```python
from build123d import *

# Parameters (mm, degrees)
FILLET1_R = 1


# Read off the part's stored shape, not the designer's step: Dog Bowl Washer
with BuildPart() as part:
    # Dog Bowl Washer outline → Dog Bowl Washer (revolve)
    with BuildSketch(Plane.XY):
        with BuildLine():
            Line((5.2705, 1.27), (6.392427617, 0))
            Line((6.392427617, 0), (12.7, 0))
            Line((12.7, 0), (12.646813167, 1.52307162))
            ThreePointArc((12.646813167, 1.52307162), (11.484828724, 4.047470654), (8.87095, 4.9911))
            Line((8.87095, 4.9911), (5.2705, 1.27))
        make_face()
    revolve(axis=Axis((0, 0, 0), (0, 1, 0)))


with BuildPart() as body_2:
    # Sketch1 → Revolve1 (revolve)
    with BuildSketch(Plane.XY, mode=Mode.PRIVATE) as revolve1_sk:
        Polygon((-14.5, 8.5), (-8.5, 8.5), (-5.5, 5.5), (-5.5, 4), (-8.5, 4), (-8.5, 0), (-14.5, 0), align=None)
    revolve(revolve1_sk.sketch.rotate(Axis((0, 10.834647468, 0), (0, -1, 0)), 270), axis=Axis((0, 10.834647468, 0), (0, -1, 0)))

    # Combine1: cut part
    add(part.part, mode=Mode.SUBTRACT)

    # Fillet1
    fillet1_edges = [body_2.edges().sort_by_distance(p)[0] for p in [
        (0, 0, -14.5),
        (0, 8.5, -8.5),
        (0, 8.5, -14.5),
    ]]
    fillet(fillet1_edges, radius=FILLET1_R)


solid = body_2.part
```
Could you check a few things on this model? Use its own coordinates, in mm. Round coordinates to 2 decimals unless told otherwise and drop trailing zeros. Order: outer loops, then holes, each group sorted by start corner. A loop starts at its lowest first (then second) coordinate and runs counter-clockwise, first axis right, second up. Notation, with made-up numbers: M 46.5,9 L 52.5,9 A13 ccw 52.5,14 Z; hole C 35.25,-8 d9. An arc over 180 degrees is marked long. One line per question, with ' | ' between items. Start each with the question number.
(1) Thinking about a two-plate mould opening in Z: for faces 1 (the face through (5, 0, -12)), 2 (the face through (5.554, 4.296, 13.394)), 3 (the face through (-5.4, 4, 1.9)), 4 (the face through (-2.743, 1.28, 12.354)), which applies, +Z half, -Z half, draft (parallel to the pull), parting line (faces both ways), or undercut?
(2) For P1, Ø1.5, axis at x = 3.5, y = 6, coming from the +Z side; P2, Ø6.5, axis at x = 0, z = 0, coming from the -Y side; P3, Ø1, axis at y = 6, z = -4, coming from the -X side; P4, Ø2, axis at x = -9, z = -10.5, coming from the +Y side, each with a flat end and sliding along its axis, tell me the tip position at first contact or that it passes through.
(3) Suppose I cut it at C-C on y = 4.5. List the corners of the cut face in (x, z) for me, then the cut area to 3 significant figures.
(4) Suppose I cut it at D-D on y = 6. List the corners of the cut face in (x, z) for me, then the cut area to 3 significant figures.
(5) Suppose I cut it at B-B on z = 0. List the corners of the cut face in (x, y) for me.
(6) Suppose I cut it at A-A on x = 0. List the corners of the cut face in (y, z) for me.
(7) Please list where these lines run through material, in increasing order: line 1 along Z through (x, y) = (-0.25, 1.25); line 2 along X through (y, z) = (4.55, 0); line 3 along X through (y, z) = (6.5, 0.75).
Geometry results:
1) face 1: draft | face 2: parting line | face 3: undercut | face 4: undercut
2) P1: z = 14.24 | P2: through | P3: x = -14.07 | P4: y = 8.5
3) outline: C 0,0 d29; C 0,0 d16.79; hole C 0,0 d21.75; hole C 0,0 d11 | area: 416 mm²
4) outline: C 0,0 d29; hole C 0,0 d12 | area: 547 mm²
5) outline: M -14.5,1 A1 ccw -13.5,0 L -12.7,0 L -12.65,1.52 A3.6 cw -8.87,4.99 L -7.91,4 L -5.5,4 L -5.5,5.5 L -8.21,8.21 A1 ccw -8.91,8.5 L -13.5,8.5 A1 ccw -14.5,7.5 Z; M 5.5,4 L 7.91,4 L 8.87,4.99 A3.6 cw 12.65,1.52 L 12.7,0 L 13.5,0 A1 ccw 14.5,1 L 14.5,7.5 A1 ccw 13.5,8.5 L 8.91,8.5 A1 ccw 8.21,8.21 L 5.5,5.5 Z
6) outline: M 0,-13.5 A1 ccw 1,-14.5 L 7.5,-14.5 A1 ccw 8.5,-13.5 L 8.5,-8.91 A1 ccw 8.21,-8.21 L 5.5,-5.5 L 4,-5.5 L 4,-7.91 L 4.99,-8.87 A3.6 cw 1.52,-12.65 L 0,-12.7 Z; M 0,12.7 L 1.52,12.65 A3.6 cw 4.99,8.87 L 4,7.91 L 4,5.5 L 5.5,5.5 L 8.21,8.21 A1 ccw 8.5,8.91 L 8.5,13.5 A1 ccw 7.5,14.5 L 1,14.5 A1 ccw 0,13.5 Z
7) line 1: -14.5 to -12.65, 12.65 to 14.5 | line 2: -14.5 to -10.79, -8.44 to -5.5, 5.5 to 8.44, 10.79 to 14.5 | line 3: -14.48 to -6.46, 6.46 to 14.48
